from build123d import *

# Parameters (mm, degrees)
SKETCH3_R               = 2.201333333
SKETCH3_R_2             = 1.693333333
BOSS_EXTRUDE1_DEPTH     = 914.4
CUT_EXTRUDE1_DEPTH      = 1473.2
CUT_EXTRUDE2_DEPTH      = 915.524310439
CUT_EXTRUDE2_DEPTH_BACK = 915.524310439
SKETCH6_R               = 3


with BuildPart() as part:
    # Sketch3 → Boss-Extrude1 (new, symmetric)
    with BuildSketch(Plane.XY):
        with BuildLine():
            Line((-1.778, 0), (-1.778, 1.27))
            ThreePointArc((-1.778, 1.27), (-1.536070654, 2.494011801), (-0.846666667, 3.533942971))
            Line((-0.846666667, 3.533942971), (2.413267273, 6.793876912))
            ThreePointArc((2.413267273, 6.793876912), (2.578074335, 6.903997469), (2.772477518, 6.942666667))
            Line((2.772477518, 6.942666667), (3.048, 6.942666667))
            ThreePointArc((3.048, 6.942666667), (3.467078619, 6.769078619), (3.640666667, 6.35))
            Line((3.640666667, 6.35), (3.640666667, 4.301066667))
            ThreePointArc((3.640666667, 4.301066667), (3.948165494, 3.558698827), (4.690533333, 3.2512))
            Line((4.690533333, 3.2512), (5.300133333, 3.2512))
            ThreePointArc((5.300133333, 3.2512), (6.042501173, 3.558698827), (6.35, 4.301066667))
            Line((6.35, 4.301066667), (6.35, 10.583333333))
            ThreePointArc((6.35, 10.583333333), (5.730042687, 12.080042687), (4.233333333, 12.7))
            Line((4.233333333, 12.7), (-4.233333333, 12.7))
            ThreePointArc((-4.233333333, 12.7), (-5.730042687, 12.080042687), (-6.35, 10.583333333))
            Line((-6.35, 10.583333333), (-6.35, 0))
            Line((-6.35, 0), (-1.778, 0))
        make_face()
        with Locations(Location((-2.116666667, 8.466666667, 0), (0, 0, 180))):
            Circle(SKETCH3_R, mode=Mode.SUBTRACT)
        with Locations(Location((3.429, 9.906, 0), (0, 0, 180))):
            Circle(SKETCH3_R_2, mode=Mode.SUBTRACT)
    extrude(amount=BOSS_EXTRUDE1_DEPTH, both=True)

    # Mirror1: part across plane


with BuildPart() as part_1:
    add(part.part)
    add(part.part.mirror(Plane.ZX))

    # Sketch5 → Cut-Extrude1 (cut)
    with BuildSketch(Plane.XY.offset(914.4)):
        with BuildLine():
            Line((-6.35, 10.583333333), (-6.35, -10.583333333))
            ThreePointArc((-6.35, -10.583333333), (-5.730042687, -12.080042687), (-4.233333333, -12.7))
            Line((-4.233333333, -12.7), (4.233333333, -12.7))
            ThreePointArc((4.233333333, -12.7), (5.730042687, -12.080042687), (6.35, -10.583333333))
            Line((6.35, -10.583333333), (6.35, -4.301066667))
            ThreePointArc((6.35, -4.301066667), (6.042501173, -3.558698827), (5.300133333, -3.2512))
            Line((5.300133333, -3.2512), (4.690533333, -3.2512))
            ThreePointArc((4.690533333, -3.2512), (3.948165494, -3.558698827), (3.640666667, -4.301066667))
            Line((3.640666667, -4.301066667), (3.640666667, -6.35))
            ThreePointArc((3.640666667, -6.35), (3.467078619, -6.769078619), (3.048, -6.942666667))
            Line((3.048, -6.942666667), (2.772477518, -6.942666667))
            ThreePointArc((2.772477518, -6.942666667), (2.578074335, -6.903997469), (2.413267273, -6.793876912))
            Line((2.413267273, -6.793876912), (-0.846666667, -3.533942971))
            ThreePointArc((-0.846666667, -3.533942971), (-1.536070654, -2.494011801), (-1.778, -1.27))
            Line((-1.778, -1.27), (-1.778, 1.27))
            ThreePointArc((-1.778, 1.27), (-1.536070654, 2.494011801), (-0.846666667, 3.533942971))
            Line((-0.846666667, 3.533942971), (2.413267273, 6.793876912))
            ThreePointArc((2.413267273, 6.793876912), (2.578074335, 6.903997469), (2.772477518, 6.942666667))
            Line((2.772477518, 6.942666667), (3.048, 6.942666667))
            ThreePointArc((3.048, 6.942666667), (3.467078619, 6.769078619), (3.640666667, 6.35))
            Line((3.640666667, 6.35), (3.640666667, 4.301066667))
            ThreePointArc((3.640666667, 4.301066667), (3.948165494, 3.558698827), (4.690533333, 3.2512))
            Line((4.690533333, 3.2512), (5.300133333, 3.2512))
            ThreePointArc((5.300133333, 3.2512), (6.042501173, 3.558698827), (6.35, 4.301066667))
            Line((6.35, 4.301066667), (6.35, 10.583333333))
            ThreePointArc((6.35, 10.583333333), (5.730042687, 12.080042687), (4.233333333, 12.7))
            Line((4.233333333, 12.7), (-4.233333333, 12.7))
            ThreePointArc((-4.233333333, 12.7), (-5.730042687, 12.080042687), (-6.35, 10.583333333))
        make_face()
    extrude(amount=-CUT_EXTRUDE1_DEPTH, mode=Mode.SUBTRACT)

    # Sketch6 → Cut-Extrude2 (cut, two sides: drawn at the far end of the back side and taken through both)
    with BuildSketch(Plane(origin=(-1.778, 0, 0), x_dir=(0, 0, -1), z_dir=(1, 0, 0)).offset(-CUT_EXTRUDE2_DEPTH_BACK)):
        with Locations(Location((901.7, 0, 0), (0, 0, 90))):
            Circle(SKETCH6_R)
        with Locations(Location((571.5, 0, 0), (0, 0, 154.954785638))):
            Circle(SKETCH6_R)
    extrude(amount=CUT_EXTRUDE2_DEPTH + CUT_EXTRUDE2_DEPTH_BACK, mode=Mode.SUBTRACT)


solid = part_1.part
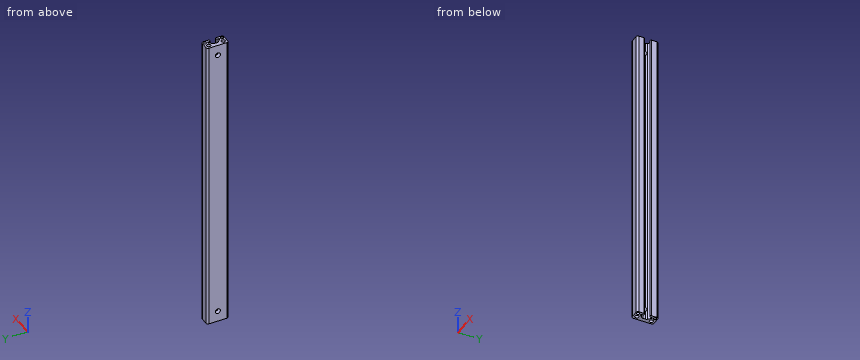
Verification items for the finished model (mm, model axes). Coordinates: 2 decimals unless noted, no trailing zeros. Answer as a JSON object with one key per item and string values.
(1) Gauge pin test, flat ends, axial feed: pin 1 Ø0.5 at (x, z) = (5, -782.5) entering from +Y; pin 2 Ø1.5 at (x, y) = (-1, 8.5) entering from +Z; pin 3 Ø1.3 at (y, z) = (-0.5, -564) entering from +X; pin 4 Ø3 at (y, z) = (-0.5, -911) entering from +X. Record the tip position at first contact, or that the pin passes through.
Report:
{"pin 1": "y = 12.64", "pin 2": "through", "pin 3": "x = -1.78", "pin 4": "x = -1.69"}
(2) Thickness scan on line 1 along Y through (x, z) = (-2.25, -778); line 2 along Y through (x, z) = (-2.75, -571.5); line 3 along Y through (x, z) = (-2.5, -767). Record the ranges inside material, lowest first.
Report:
{"line 1": "-12.7 to -10.66, -6.27 to 6.27, 10.66 to 12.7", "line 2": "-12.7 to -10.57, -6.36 to -3, 3 to 6.36, 10.57 to 12.7", "line 3": "-12.7 to -10.63, -6.3 to 6.3, 10.63 to 12.7"}
(3) Cross-section at A-A on z = -610. Give the number of separate pieces and of enclosed holes in the cut face, plus the area to 3 significant figures.
Report:
{"separate pieces": "1", "enclosed holes": "4", "area": "196 mm^2"}
